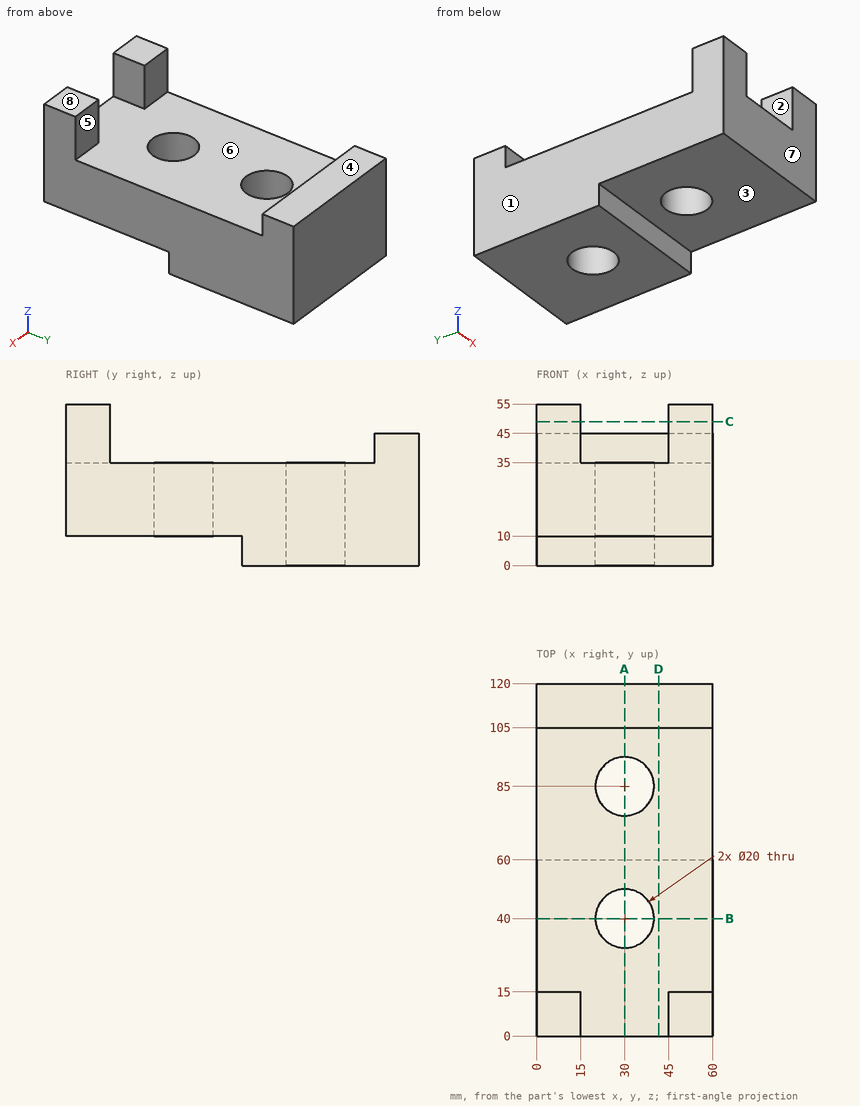
Print and shaded views of the part. All mm, measured from the part's lowest x, y and z. A direction names the side the tool comes from. Give positions to 0.01 mm unless a question says otherwise; leave off trailing zeros. Write each loop counter-clockwise with the first axis right and the second up, starting at its lowest first coordinate (ties: lowest second). Pieces come first, ordered by that corner, then holes. Notation, with made-up numbers: (-8.75, 63.5) -> (7.25, 63.5) arc R21 ccw to (7.25, 71.5) -> close; hole circle Ø4 at (80, 62.25). An arc over 180 degrees is marked (long way). Write each question's results on one line, items separated by ' | '.
1. Which spindle directions (+Z, -Z, +X, -X, +Y, -Y) get a long thin tool onto all of the face, cutting with end or side? Do the marked faces 1, 2, 3, 4 and 5. Say none if no direction does.
Geometry check:
face 1: +Z, -Z, -X, +Y, -Y | face 2: +Z, -Y | face 3: -Z, +X, -X, -Y | face 4: +Z, +X, -X, +Y | face 5: +Z, +X, -X
2. Two-plate mould, pull along Y, no slides. Class the marked faces 6, 7 and 8: pulls with the +Y half, pulls with the -Y half, needs draft (parallel to the pull), parting line crosses it, or undercut.
Geometry check:
face 6: undercut | face 7: pulls with the -Y half | face 8: needs draft
3. Cut at B-B, the plane y = 40. Write the cut outline in (x, z).
Geometry check:
outline: (0, 10) -> (20, 10) -> (20, 35) -> (0, 35) -> close; (40, 10) -> (60, 10) -> (60, 35) -> (40, 35) -> close
4. Cut at C-C, the plane z = 49. Write the cut outline in (x, y), then the cut area to 3 significant figures.
Geometry check:
outline: (0, 0) -> (15, 0) -> (15, 15) -> (0, 15) -> close; (45, 0) -> (60, 0) -> (60, 15) -> (45, 15) -> close | area: 450 mm²
5. Cut at A-A, the plane x = 30. Write the cut outline in (y, z).
Geometry check:
outline: (0, 10) -> (30, 10) -> (30, 35) -> (0, 35) -> close; (50, 10) -> (60, 10) -> (60, 0) -> (75, 0) -> (75, 35) -> (50, 35) -> close; (95, 0) -> (120, 0) -> (120, 45) -> (105, 45) -> (105, 35) -> (95, 35) -> close
6. Drop flat-ended pins along their axis: P1, Ø12, axis at x = 25, y = 110, coming from the +Z side; P2, Ø4, axis at x = 12.5, y = 50.5, coming from the +Z side; P3, Ø16, axis at x = 30, y = 85, coming from the +Z side; P4, Ø1.5, axis at x = 8, y = 41.5, coming from the -Z side. Give the stop position or say it passes through.
Geometry check:
P1: z = 45 | P2: z = 35 | P3: through | P4: z = 10
7. Wall check: probe 1 along Y at (x, z) = (30, 32.5); probe 2 along X at (y, z) = (11.5, 44); probe 3 along Y at (x, z) = (38, 22). Give the ranges that are in metal, low to high. Write a range as [from, to].
Geometry check:
probe 1: [0, 30], [50, 75], [95, 120] | probe 2: [0, 15], [45, 60] | probe 3: [0, 34], [46, 79], [91, 120]
8. Cut at D-D, the plane x = 41.5. Write the cut outline in (y, z).
Geometry check:
outline: (0, 10) -> (60, 10) -> (60, 0) -> (120, 0) -> (120, 45) -> (105, 45) -> (105, 35) -> (0, 35) -> close
